Autodesk Fusion 360 part; units mm, degrees
sketch "Boceto2" plane through (0, 0, 0) normal (0, 1, 0) x (1, 0, 0)
  line L0 (7.5, 0) -> (9.2213, 0)
  line L1 (14.5, -80.7) -> (7.5, -80.7)
  line L2 (0, -73.2) -> (0, -7.5)
  arc A0 (0, -73.2) -> (7.5, -80.7) centre (7.5, -73.2) ccw
  arc A1 (7.5, 0) -> (0, -7.5) centre (7.5, -7.5) ccw
  line L3 (12.7, -78.7828) -> (7.5, -78.7828)
  arc A2 (1.9172, -73.2) -> (7.5, -78.7828) centre (7.5, -73.2) ccw
  line L4 (7.5, -3.5523) -> (7.5, -2.6)
  line L5 (7.5, -2.6) -> (6.3, -2.6)
  line L6 (6.3, -2.6) -> (6.3, -9.6)
  line L7 (6.3, -9.6) -> (7.5, -9.6)
  line L8 (7.5, -9.6) -> (7.5, -8.5)
  line L9 (9.2213, -8.5) -> (9.2213, -10.6)
  line L10 (8.7213, -11.1) -> (4.9, -11.1)
  line L11 (4.4, -10.6) -> (4.4, -5.7)
  arc A3 (4.4, -5.7) -> (2.8546, -5.0381) centre (3.3076, -6.1153) ccw
  arc A4 (4.4, -5.7) -> (2.1854, -5.7893) centre (3.3076, -6.1153) ccw
  arc A5 (2.1854, -5.7893) -> (1.9172, -7.5) centre (7.5062, -7.5) ccw
  arc A6 (9.2213, -8.5) -> (7.5, -8.5) centre (8.3607, -9.2707) ccw
  arc A7 (7.5, -3.5523) -> (9.2213, -3.5523) centre (8.3607, -3.072) ccw
  line L12 (9.2213, -3.5523) -> (9.2213, 0)
  line L13 (20.1126, -1.9172) -> (20.115, -1.9172)
  line L14 (1.9172, -21.6025) -> (7.2, -21.6025)
  line L15 (7.7, -22.1025) -> (7.7, -23)
  line L16 (7.2, -23.5) -> (1.9172, -23.5)
  line L17 (1.9172, -45.6046) -> (20.0634, -45.6046)
  line L18 (20.0634, -43.7426) -> (20.0634, -43.7426)
  line L19 (20.036, -60.0002) -> (20.036, -60.0234)
  line L20 (20.036, -61.8138) -> (3.4172, -61.8138)
  line L21 (14.5, -80.7) -> (14.5, -78.7828)
  line L22 (1.9172, -21.6025) -> (1.9172, -7.5)
  arc A8 (7.2, -23.5) -> (7.7, -23) centre (7.2, -23) ccw
  arc A9 (7.7, -22.1025) -> (7.2, -21.6025) centre (7.2, -22.1025) ccw
  line L23 (1.9172, -42.2426) -> (1.9172, -23.5)
  arc A10 (1.9172, -42.2426) -> (3.4172, -43.7426) centre (3.4172, -42.2426) ccw
  line L24 (6.2895, -43.7426) -> (6.2895, -43.415)
  line L25 (4.4317, -43.415) -> (4.4317, -43.7426)
  arc A11 (6.2895, -43.415) -> (4.4317, -43.415) centre (5.3606, -43.415) ccw
  line L26 (20.0634, -43.7426) -> (6.2895, -43.7426)
  line L27 (4.4317, -43.7426) -> (3.4172, -43.7426)
  line L28 (1.9172, -73.2) -> (1.9172, -63.3138)
  line L29 (1.9172, -60.0002) -> (1.9172, -45.6046)
  arc A12 (3.4172, -61.8138) -> (1.9172, -63.3138) centre (3.4172, -63.3138) ccw
  line L30 (12.9, -78.5828) -> (12.9, -78.2)
  line L31 (14.5, -78.2) -> (14.5, -78.7828)
  arc A13 (14.5, -78.2) -> (12.9, -78.2) centre (13.7, -78.34) ccw
  arc A14 (4.4, -10.6) -> (4.9, -11.1) centre (4.9, -10.6) ccw
  arc A15 (8.7213, -11.1) -> (9.2213, -10.6) centre (8.7213, -10.6) ccw
  arc A16 (12.7, -78.7828) -> (12.9, -78.5828) centre (12.7, -78.5828) ccw
  line L32 (32.4735, -22.1342) -> (32.4712, -23.0317)
  line L33 (35.8029, -10.6401) -> (35.8154, -5.7401)
  arc A17 (36.701, -43.7851) -> (38.2048, -42.289) centre (36.7048, -42.2851) ccw
  line L34 (38.1594, -60.0465) -> (38.1962, -45.651)
  line L35 (33.8286, -43.7778) -> (33.8295, -43.4502)
  arc A18 (35.6873, -43.4549) -> (33.8295, -43.4502) centre (34.7584, -43.4526) ccw
  line L36 (32.7209, -3.5846) -> (32.7233, -2.6322)
  line L37 (35.6864, -43.7825) -> (36.701, -43.7851)
  line L38 (32.9699, -23.5329) -> (38.2527, -23.5464)
  line L39 (40.0429, -73.2512) -> (40.2108, -7.5514)
  line L40 (38.2048, -42.289) -> (38.2527, -23.5464)
  arc A19 (32.4712, -23.0317) -> (32.9699, -23.5329) centre (32.9712, -23.0329) ccw
  line L41 (35.6873, -43.4549) -> (35.6864, -43.7825)
  arc A20 (37.3625, -5.0822) -> (35.8154, -5.7401) centre (36.9067, -6.1583) ccw
  line L42 (30.9869, -8.5278) -> (30.9816, -10.6278)
  line L43 (27.1292, -78.601) -> (27.1301, -78.2182)
  arc A21 (38.2936, -7.5465) -> (38.0298, -5.8351) centre (32.7046, -7.5322) ccw
  line L44 (25.5301, -78.2141) -> (25.5286, -78.7969)
  line L45 (32.73, -0.0322) -> (31.0086, -0.0278)
  arc A22 (40.2108, -7.5514) -> (32.73, -0.0322) centre (32.7108, -7.5322) ccw
  arc A23 (35.3016, -11.1388) -> (35.8029, -10.6401) centre (35.3029, -10.6388) ccw
  arc A24 (32.5237, -80.732) -> (40.0429, -73.2512) centre (32.5429, -73.232) ccw
  arc A25 (32.9748, -21.6355) -> (32.4735, -22.1342) centre (32.9735, -22.1355) ccw
  line L46 (32.7054, -9.6322) -> (32.7082, -8.5322)
  arc A26 (30.9816, -10.6278) -> (31.4803, -11.1291) centre (31.4816, -10.6291) ccw
  line L47 (33.9233, -2.6353) -> (33.9054, -9.6353)
  line L48 (27.3286, -78.8015) -> (32.5286, -78.8148)
  arc A27 (38.0298, -5.8351) -> (35.8154, -5.7401) centre (36.9067, -6.1583) ccw
  arc A28 (38.151, -63.3601) -> (36.6548, -61.8563) centre (36.651, -63.3563) ccw
  arc A29 (30.9996, -3.5802) -> (32.7209, -3.5846) centre (31.8615, -3.102) ccw
  line L49 (30.9996, -3.5802) -> (31.0086, -0.0278)
  arc A30 (32.5286, -78.8148) -> (38.1257, -73.2463) centre (32.5429, -73.232) ccw
  line L50 (38.1257, -73.2463) -> (38.151, -63.3601)
  line L51 (38.2576, -21.649) -> (38.2936, -7.5465)
  line L52 (31.4803, -11.1291) -> (35.3016, -11.1388)
  line L53 (25.5237, -80.7141) -> (25.5286, -78.7969)
  arc A31 (27.1292, -78.601) -> (27.3286, -78.8015) centre (27.3292, -78.6015) ccw
  line L54 (32.7233, -2.6322) -> (33.9233, -2.6353)
  line L55 (33.9054, -9.6353) -> (32.7054, -9.6322)
  arc A32 (32.7082, -8.5322) -> (30.9869, -8.5278) centre (31.8456, -9.3007) ccw
  line L56 (38.2576, -21.649) -> (32.9748, -21.6355)
  line L57 (25.5237, -80.7141) -> (32.5237, -80.732)
  arc A33 (27.1301, -78.2182) -> (25.5301, -78.2141) centre (26.3298, -78.3561) ccw
  line L58 (20.0548, -43.7426) -> (33.8286, -43.7778)
  line L59 (38.1962, -45.651) -> (20.05, -45.6046)
  line L60 (20.036, -61.8138) -> (36.6548, -61.8563)
  line L61 (1.9172, -60.0002) -> (38.1594, -60.0465)
  line L62 (20.036, -61.8138) -> (20.0119, -80.7) construction
  line L63 (20.115, 0) -> (20.0591, -43.7426) construction
  line L64 (20.0567, -45.6046) -> (20.0383, -60.0234) construction
  point P0 (0, -80.7)
  point P1 (40.0237, -80.7511)
  point P2 (40.2299, -0.0514)
  point P3 (40.2299, -0.0514)
  dimension "d10" = 80.7
  dimension "d12" = 7.5
  dimension "d14" = 0.5
  dimension "d15" = 1.5
  dimension "d16" = 1.5
  dimension "d17" = 0.5
  dimension "d18" = 0.2
extrude "Extruir1" add sketch "Boceto2" along normal blind 10
Source: CAD feature listing. Evaluate the final solid. Frame: model axes, mm. A direction names the side the tool comes from. Round coordinates to 2 decimals unless told otherwise and drop trailing zeros. Write each loop counter-clockwise with the first axis right and the second up, starting at its lowest first coordinate (ties: lowest second). Pieces come first, ordered by that corner, then holes. Notation, with made-up numbers: M -1,-0.75 L 52,-0.75 A18 ccw 52,33.25 Z; hole C 26.25,14 d7. An arc over 180 degrees is marked long. Answer as a JSON object with one key per item and string values. Group by question number.
(1) Section query B-B on z = 16.5. Output: boundary loops of the cut face in (x, y), then the cut area to 3 significant figures.
(2) Ray query, line 1 (Z direction, x = 11.5, y = 7.5); line 2 (Z direction, x = 16, y = 7.5); line 3 (Z direction, x = 2.5, y = 6.25). Return the intervals inside material, ascending. Write a range as [from, to].
(3) Reachability of faces 4 (the flat face through (14.5, 5, 79)), 5 (the flat face through (13, 5, 43.743)) from +Z, -Z, +X, -X, +Y, -Y: full face, straight path, thin tool, end or side. Return the list, or none.
(4) Section query A-A on x = 24.5. Output: boundary loops of the cut face in (y, z).
(5) Mould query, pull axis Z, two halves, no side actions, for faces 1 (the cylindrical face through (34.74, 4.93, 42.524)), 2 (the flat face through (9.221, 5, 10)), 3 (the cylindrical face through (2.255, 4.93, 78.561)). Classes: +Z half, -Z half, draft (parallel to the pull), parting line (faces both ways), or undercut.
(6) First-contact query: pin 1 (4 mm diameter, centred on y = 7.5, z = 1.5, fed in from +X); pin 2 (3.5 mm diameter, centred on y = 6.5, z = 5.5, fed in from +X); pin 3 (3 mm diameter, centred on y = 3.5, z = 34, fed in from +X). Flat tips, straight axial feed; report the tip coordinate or a pass-through.
Computed values:
{
 "1": {"outline": "M 0,0 L 1.92,0 L 1.92,10 L 0,10 Z; M 38.27,0 L 40.19,0 L 40.19,10 L 38.27,10 Z", "area": "38.3 mm^2"},
 "2": {"line 1": "[43.74, 45.6], [60.01, 61.81], [78.78, 80.7]", "line 2": "[43.74, 45.6], [60.02, 61.81]", "line 3": "[1.91, 5.27], [21.6, 23.5], [43.43, 45.6], [60, 62.13], [75.68, 78.79]"},
 "3": {"face 4": "+Z, +Y, -Y", "face 5": "+Y, -Y"},
 "4": {"outline": "M 0,43.75 L 10,43.75 L 10,45.62 L 0,45.62 Z; M 0,60.03 L 10,60.03 L 10,61.83 L 0,61.83 Z"},
 "5": {"face 1": "undercut", "face 2": "draft", "face 3": "+Z half"},
 "6": {"pin 1": "x = 39.03", "pin 2": "x = 40.21", "pin 3": "x = 40.15"}
}
